Model file for the job. Use its own axes, mm. Face numbers are marked on the shaded views. A direction names the side the tool comes from. Round coordinates to 2 decimals unless told otherwise and drop trailing zeros. Write each loop counter-clockwise with the first axis right and the second up, starting at its lowest first coordinate (ties: lowest second). Pieces come first, ordered by that corner, then holes.
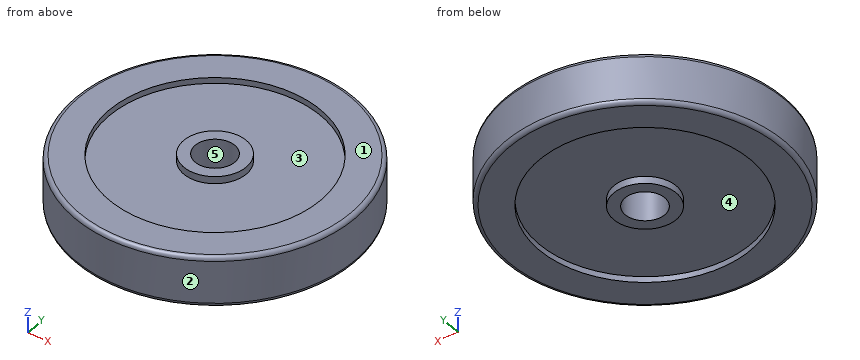
```python
from build123d import *

# Parameters (mm, degrees)
SKETCH1_W = 15
SKETCH1_H = 75.965253598
FILLET1_R = 3


with BuildPart() as part:
    # Sketch1 → Revolve1 (revolve)
    with BuildSketch(Plane(origin=(0, 0, 0), x_dir=(0, 0, -1), z_dir=(1, 0, 0)), mode=Mode.PRIVATE) as revolve1_sk:
        Polygon((19.7, 14.7), (-19.7, 14.7), (-19.7, 23.2), (-14.4, 23.2), (-14.4, 78.4), (-18.7, 78.4), (-18.7, 103.6), (18.7, 103.6), (18.7, 78.4), (14.4, 78.4), (14.4, 23.2), (19.7, 23.2), align=None)
        with Locations((0, 60.876891385)):
            Rectangle(SKETCH1_W, SKETCH1_H, mode=Mode.SUBTRACT)
    revolve(revolve1_sk.sketch.rotate(Axis((0, 0, 15.387931034), (0, 0, -1)), 90), axis=Axis((0, 0, 15.387931034), (0, 0, -1)))

    # Fillet1
    fillet1_edges = [part.edges().sort_by_distance(p)[0] for p in [
        (-103.6, 0, -18.7),
        (-103.6, 0, 18.7),
    ]]
    fillet(fillet1_edges, radius=FILLET1_R)


solid = part.part
```
1) Cut at A-A on x = 0. Give the number of separate pieces and of enclosed holes in the cut face, and give its area (3 significant figures).
2) Flat gauge pins, fed straight in: pin 1 Ø1.5 at (y, z) = (75.5, -14.5) entering from -X; pin 2 Ø1.5 at (y, z) = (62, 8) entering from +X; pin 3 Ø5 at (y, z) = (-77.5, 13) entering from -X. Where does each tip first touch, or does it go through?
3) Which spindle directions (+Z, -Z, +X, -X, +Y, -Y) get a long thin tool onto all of the face, cutting with end or side? Do the marked faces 4 and 5. Say none if no direction does.
4) Cut at B-B on z = 4. List the corners of the cut face in (x, y).
5) Pull direction X, two halves, no side cores. Call the marked faces 1, 2 and 3: released by +X, released by -X, zero draft, split by the parting line, or undercut.
6) Wall check: probe 1 along Y at (x, z) = (0, 6); probe 2 along Y at (x, z) = (0, -16); probe 3 along Y at (x, z) = (-18.5, 16.5). Give the ranges that are in metal, low to high.
7) Cut at D-D on z = -12. List the corners of the cut face in (x, y).
Result sheet:
1. separate pieces: 2
1. enclosed holes: 2
1. area: 3,450 mm2
2. pin 1: stops at x = -71.73
2. pin 2: stops at x = 83.55
2. pin 3: stops at x = -71.47
3. face 4: -Z
3. face 5: +Z, -Z
4. outline: circle Ø207.2 at (0, 0); circle Ø45.79 at (0, 0); hole circle Ø197.72 at (0, 0); hole circle Ø29.4 at (0, 0)
5. face 1: zero draft
5. face 2: split by the parting line
5. face 3: undercut
6. probe 1: y = -103.6 to -98.86, -22.89 to -14.7, 14.7 to 22.89, 98.86 to 103.6
6. probe 2: y = -103.58 to -78.4, -23.2 to -14.7, 14.7 to 23.2, 78.4 to 103.58
6. probe 3: y = -101.82 to -76.19, -14 to 14, 76.19 to 101.82
7. outline: circle Ø207.2 at (0, 0); hole circle Ø29.4 at (0, 0)
